Source: three-view drawing plus pictorial views. Frame: mm from the lowest corner of the part. A direction names the side the tool comes from. Coordinates: 2 decimals unless noted, no trailing zeros. Loops run counter-clockwise (first coordinate to the right, second up) from the corner with the lowest first, then second, coordinate; pieces in that order, holes last. Notation, with made-up numbers: M 48.25,-39 L 53.25,-39 A19 cw 53.25,-9 Z; hole C 46.25,-38.75 d5. An arc over 180 degrees is marked long. Write each question's results on one line, items separated by ' | '. Start each with the question number.
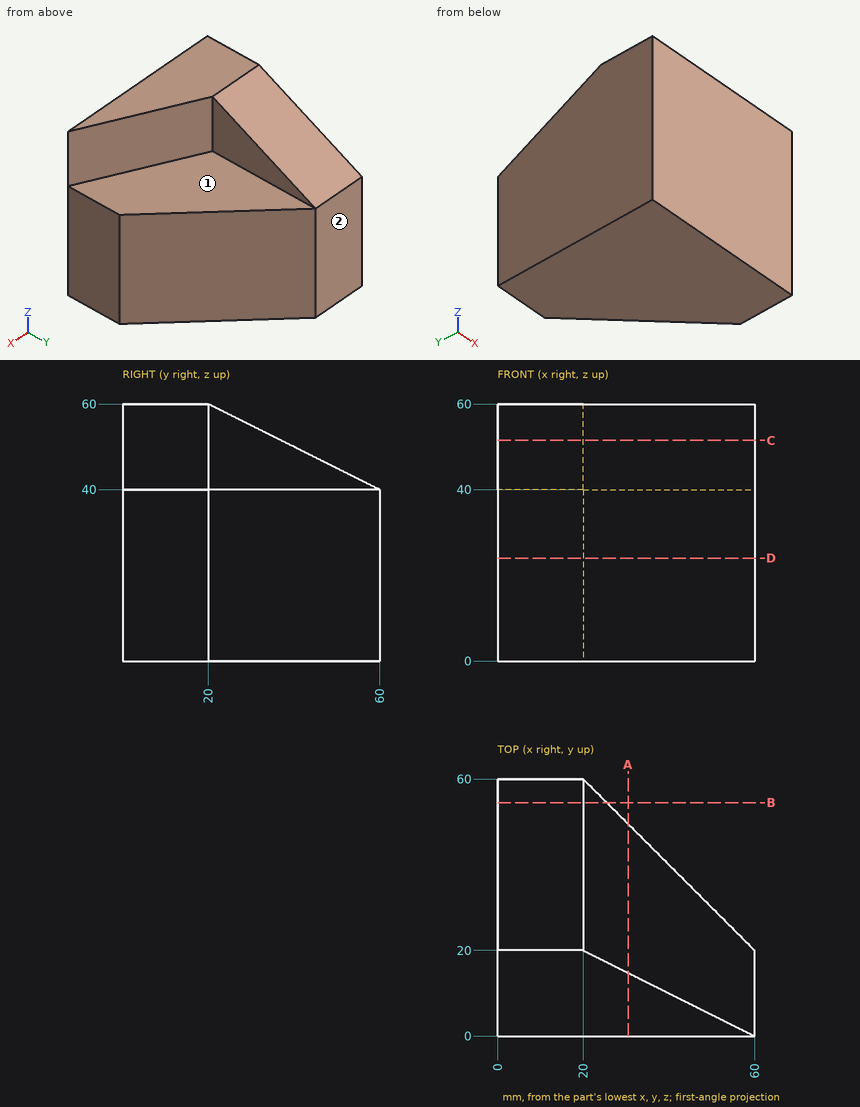
Item 1: Contact query for flat-ended pins moving along their axis: P1, Ø6, axis at x = 36.5, y = 26.5, coming from the -Z side; P2, Ø6, axis at x = 50, y = 19.5, coming from the +Z side; P3, Ø12, axis at x = 49.5, z = 53, coming from the +Y side; P4, Ø3, axis at y = 51.5, z = 21.5, coming from the +X side. Output: stop coordinate, or through.
Item 2: Set-up query: the marked faces 1 and 2. Return all of +Z, -Z, +X, -X, +Y, -Y with unobstructed straight access to the full face (end or side cutting, diameter ignored); none if empty.
Item 3: Section C-C, the plane z = 51.5. Return loops of the section in (x, y).
Item 4: Ray query, L1, parallel to X at y = 53, z = 35; L2, parallel to X at y = 23.5, z = 36.5; L3, parallel to Y at x = 38, z = 18.5. Return the intervals inside material, ascending. Write a range as [from, to].
Item 5: Section D-D, the plane z = 24. Return loops of the section in (x, y).
Item 6: Section A-A, the plane x = 30.5. Return loops of the section in (y, z), plus the area to 4 significant figures.
Item 7: Section B-B, the plane y = 54.5. Return loops of the section in (x, z), plus the area to 4 significant figures.
Solutions:
1) P1: stops at z = 0 | P2: stops at z = 40 | P3: stops at y = 8.25 | P4: stops at x = 30
2) face 1: +Z, +X, +Y | face 2: +Z, -Z, +X, -X, +Y
3) outline: M 0,0 L 60,0 L 20,20 L 20,37 L 0,37 Z
4) L1: x = [0, 27] | L2: x = [0, 56.5] | L3: y = [0, 42]
5) outline: M 0,0 L 60,0 L 60,20 L 20,60 L 0,60 Z
6) outline: M 0,0 L 49.5,0 L 49.5,40 L 14.75,40 L 14.75,60 L 0,60 Z | area: 2,275 mm²
7) outline: M 0,0 L 25.5,0 L 25.5,40 L 20,40 L 20,42.75 L 0,42.75 Z | area: 1,075 mm²
